Geometry check sheet. Reference: the model listing, model coordinates, mm. A direction names the side the tool comes from. Give positions to 0.01 mm unless a question says otherwise; leave off trailing zeros. Write each loop counter-clockwise with the first axis right and the second up, starting at its lowest first coordinate (ties: lowest second). Pieces come first, ordered by that corner, then holes. Notation, with made-up numbers: (83, 11.5) - (99, 11.5) arc R12 ccw to (99, 17.5) - close; hole circle Ø10 at (-36.75, 83.25). An arc over 180 degrees is marked (long way). Write item = value, one per line. Start each with the question number.
(1) Thickness scan on L1, parallel to Z at x = -139, y = 3; L2, parallel to Z at x = -105, y = 2.25. Record the ranges inside material, lowest first.
(2) Depth check by flat-ended pin: pin 1 Ø2 at (x, y) = (-3, 4) entering from +Z; pin 2 Ø4 at (x, y) = (-84, 5.5) entering from +Z; pin 3 Ø1.5 at (x, y) = (-1, 5.5) entering from +Z; pin 4 Ø4 at (y, z) = (11.5, 21) entering from +X. Enter the tip coordinate at first touch or a pass-through.
(3) Section check C-C, the plane y = 10.75. Enter the section's corners in (x, z).
(4) Access from +Z, -Z, +X, -X, +Y, -Y to the whole of each face (thin tool, end or side, straight path). Record for faces 4 (the flat face through (-1.4, 6, 43)), 5 (the flat face through (-11.589, 6.11, 7.056)), 6 (the flat face through (-2, 4, 12.8)).
(5) Section check B-B, the plane x = -31. Enter the section's corners in (y, z), plus the area to 3 significant figures.
(6) Section check A-A, the plane z = 36.5. Enter the section's corners in (x, y), plus the area to 3 significant figures.
(7) Draft check along Y on faces 1 (the flat face through (0, 5, 22)), 2 (the flat face through (-2, 2.6, 29)), 3 (the flat face through (-63, 8, 26)). Enter one of: pulls with the +Y half, pulls with the -Y half, needs draft (parallel to the pull), parting line crosses it, or undercut.
```python
from build123d import *

# Parameters (mm, degrees)
P_IDAT_VYSUNUT_M1_DEPTH  = 8
SKICA3_W                 = 1.4
SKICA3_H                 = 2.8
ODEBRAT_VYSUNUT_M1_DEPTH = 4.4
P_IDAT_START             = 8
SKICA5_W                 = 16
SKICA5_H                 = 8
P_IDAT_VYSUNUT_M2_DEPTH  = 16
ODEBRAT_VYSUNUT_M3_DEPTH = 161.57934176
ODEBRAT_VYSUNUT_M4_DEPTH = 161.57934176
SKICA4_W                 = 2.8
SKICA4_H                 = 2.8
ODEBRAT_VYSUNUT_M2_DEPTH = 4.4


with BuildPart() as part:
    # Skica2 → Přidat vysunutím1 (new body)
    with BuildSketch(Plane(origin=(0, 0, 0), x_dir=(1, 0, 0), z_dir=(0, 1, 0))):
        Polygon((0, 0), (0, -55.45), (-149.85, -3), (-127.147799643, -3), (-107, -10.052066008), (-107, 0), (-92, 0), (-92, -15.302316258), (-7.3, -44.948729338), (-7.3, 0), align=None)
    extrude(amount=P_IDAT_VYSUNUT_M1_DEPTH)

    # Skica3 → Odebrat vysunutím1 (cut)
    with BuildSketch(Plane(origin=(0, 8, 0), x_dir=(1, 0, 0), z_dir=(0, 1, 0))):
        with Locations((-0.7, -43)):
            Rectangle(SKICA3_W, SKICA3_H)
    extrude(amount=-ODEBRAT_VYSUNUT_M1_DEPTH, mode=Mode.SUBTRACT)

    # Skica5 → Přidat vysunutím2 (add)
    with BuildSketch(Plane(origin=(0, 8, 0), x_dir=(1, 0, 0), z_dir=(0, 1, 0)).offset(P_IDAT_START)):
        with Locations((-8, -7)):
            Rectangle(SKICA5_W, SKICA5_H)
    extrude(amount=-P_IDAT_VYSUNUT_M2_DEPTH)

    # Skica6 → Odebrat vysunutím3 (cut, through all)
    with BuildSketch(Plane(origin=(0, 0, 0), x_dir=(0, 0, -1), z_dir=(1, 0, 0))):
        Polygon((-11, 8), (-11, 16), (-3, 16), align=None)
    extrude(amount=-ODEBRAT_VYSUNUT_M3_DEPTH, mode=Mode.SUBTRACT)

    # Skica7 → Odebrat vysunutím4 (cut, through all)
    with BuildSketch(Plane.XZ):
        Polygon((-16, 3), (-16, 11), (-7.3, 11), align=None)
    extrude(amount=-ODEBRAT_VYSUNUT_M4_DEPTH, mode=Mode.SUBTRACT)

    # Skica4 → Odebrat vysunutím2 (cut)
    with BuildSketch(Plane(origin=(0, 0, 0), x_dir=(0, 0, -1), z_dir=(1, 0, 0))):
        with Locations((-47, 4)):
            Rectangle(SKICA4_W, SKICA4_H)
        with Locations((-29.2, 4)):
            Rectangle(SKICA4_W, SKICA4_H)
        with Locations((-11.4, 4)):
            Rectangle(SKICA4_W, SKICA4_H)
    extrude(amount=-ODEBRAT_VYSUNUT_M2_DEPTH, mode=Mode.SUBTRACT)


solid = part.part
```
Model answer:
q1.L1 = 3 to 6.8
q1.L2 = 0 to 18.7
q2.pin_1 = 54.75
q2.pin_2 = 26.75
q2.pin_3 = 55.36
q2.pin_4 = through
q3.outline = (-16, 3) - (0, 3) - (0, 8.25) - (-10.29, 8.25) - close
q4.face_4 = +X, +Y
q4.face_5 = +Y, -Y
q4.face_6 = +X
q5.outline = (0, 36.65) - (8, 36.65) - (8, 44.6) - (0, 44.6) - close
q5.area = 63.6 mm²
q6.outline = (-54.14, 0) - (-31.44, 0) - (-31.44, 8) - (-54.14, 8) - close; (-7.3, 0) - (0, 0) - (0, 8) - (-7.3, 8) - close
q6.area = 240 mm²
q7.face_1 = needs draft
q7.face_2 = undercut
q7.face_3 = pulls with the +Y half
